```python
from build123d import *

# Parameters (mm, degrees)
BOSS_EXTRUDE1_DEPTH       = 5
M3X0_5_TAPPED_HOLE1_D     = 2.5
M3X0_5_TAPPED_HOLE1_DEPTH = 3
M3X0_5_TAPPED_HOLE1_TIP   = 0.751075774
BOSS_EXTRUDE2_DEPTH       = 5
CUT_EXTRUDE1_DEPTH        = 6
BOSS_EXTRUDE3_DEPTH       = 5
SKETCH12_W                = 42.426406872
SKETCH12_H                = 0.46
BOSS_EXTRUDE4_DEPTH       = 5
SKETCH13_W                = 0.46
SKETCH13_H                = 42.886406871
BOSS_EXTRUDE5_DEPTH       = 5
M2X0_4_TAPPED_HOLE1_D     = 1.6
SKETCH20_W                = 42.886406872
SKETCH20_H                = 1.7
CUT_EXTRUDE2_DEPTH        = 6
M3X0_5_TAPPED_HOLE3_D     = 2.5
M3X0_5_TAPPED_HOLE3_DEPTH = 6
M3X0_5_TAPPED_HOLE3_TIP   = 0.751075774


with BuildPart() as part:
    # Sketch2 → Boss-Extrude1 (new body)
    with BuildSketch(Plane.XY):
        Polygon((-19.445436483, 19.445436483), (26.516504294, -26.516504294), (-19.445436483, -26.516504294), align=None)
    extrude(amount=BOSS_EXTRUDE1_DEPTH)

    # M3x0.5 Tapped Hole1
    with Locations(Plane(origin=(0, 0, 0), x_dir=(0, 0, -1), z_dir=(0.707106781, 0.707106781, 0))):
        with Locations((-2.75, 19.75), (-2.75, -29.75)):
            Hole(M3X0_5_TAPPED_HOLE1_D / 2, depth=M3X0_5_TAPPED_HOLE1_DEPTH)
            with Locations((0, 0, -(M3X0_5_TAPPED_HOLE1_DEPTH + M3X0_5_TAPPED_HOLE1_TIP / 2))):  # 118° drill point
                Cone(0, M3X0_5_TAPPED_HOLE1_D / 2, M3X0_5_TAPPED_HOLE1_TIP, mode=Mode.SUBTRACT)

    # Sketch6 → Boss-Extrude2 (add, through all)
    with BuildSketch(Plane.XY.offset(5)):
        Polygon((-19.445436483, 19.445436483), (-15.909902577, 15.909902577), (-14.495689014, 17.324116139), (-18.03122292, 20.859650045), align=None)
        Polygon((26.516504294, -26.516504294), (22.980970389, -22.980970389), (24.395183951, -21.566756826), (27.930717857, -25.102290732), align=None)
    extrude(amount=-BOSS_EXTRUDE2_DEPTH)

    # Sketch7 → Cut-Extrude1 (cut, through all)
    with BuildSketch(Plane.XY.offset(5)):
        Polygon((-18.03122292, 20.859650045), (-14.495689014, 17.324116139), (-19.445436483, 12.374368671), (-19.445436483, 19.445436483), align=None)
        Polygon((24.395183951, -21.566756826), (19.445436483, -26.516504294), (26.516504294, -26.516504294), (27.930717857, -25.102290732), align=None)
    extrude(amount=-CUT_EXTRUDE1_DEPTH, mode=Mode.SUBTRACT)

    # Sketch11 → Boss-Extrude3 (add, through all)
    with BuildSketch(Plane(origin=(0, 0, 0), x_dir=(-1, 0, 0), z_dir=(0, 0, -1))):
        Polygon((-19.445436483, -26.516504294), (-22.980970389, -26.516504294), (-22.980970389, -22.980970389), align=None)
        Polygon((19.445436483, 12.374368671), (19.445436483, 15.909902577), (15.909902577, 15.909902577), align=None)
    extrude(amount=-BOSS_EXTRUDE3_DEPTH)

    # Sketch12 → Boss-Extrude4 (add, through all)
    with BuildSketch(Plane.XY.offset(5)):
        with Locations((1.767766953, -26.746504294)):
            Rectangle(SKETCH12_W, SKETCH12_H)
    extrude(amount=-BOSS_EXTRUDE4_DEPTH)

    # Sketch13 → Boss-Extrude5 (add, through all)
    with BuildSketch(Plane.XY.offset(5)):
        with Locations((-19.675436483, -5.533300859)):
            Rectangle(SKETCH13_W, SKETCH13_H)
    extrude(amount=-BOSS_EXTRUDE5_DEPTH)

    # M2x0.4 Tapped Hole1 (through all)
    with Locations(Plane(origin=(0, 0, 0), x_dir=(-1, 0, 0), z_dir=(0, 0, -1))):
        with Locations((17.905436483, -11.976504294), (17.905436483, -21.976504294)):
            Hole(M2X0_4_TAPPED_HOLE1_D / 2)

    # Sketch20 → Cut-Extrude2 (cut, through all)
    with BuildSketch(Plane.XY.offset(5)):
        with Locations((1.537766953, -26.126504294)):
            Rectangle(SKETCH20_W, SKETCH20_H)
    extrude(amount=-CUT_EXTRUDE2_DEPTH, mode=Mode.SUBTRACT)

    # M3x0.5 Tapped Hole3
    with Locations(Plane(origin=(0, -25.276504294, 0), x_dir=(-1, 0, 0), z_dir=(0, -1, 0))):
        with Locations((7.905436483, -2.5), (-7.094563517, -2.5)):
            Hole(M3X0_5_TAPPED_HOLE3_D / 2, depth=M3X0_5_TAPPED_HOLE3_DEPTH)
            with Locations((0, 0, -(M3X0_5_TAPPED_HOLE3_DEPTH + M3X0_5_TAPPED_HOLE3_TIP / 2))):  # 118° drill point
                Cone(0, M3X0_5_TAPPED_HOLE3_D / 2, M3X0_5_TAPPED_HOLE3_TIP, mode=Mode.SUBTRACT)


solid = part.part
```
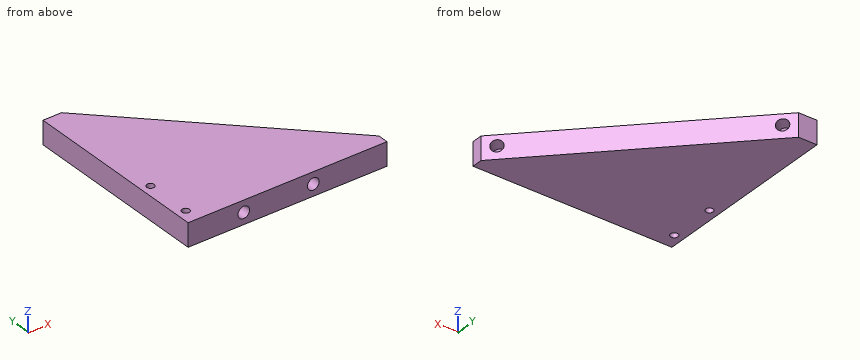
Read the model definition and answer for the solid it produces. Units are mm, in the model's axes. Coordinates: 2 decimals unless noted, no trailing zeros. Order: outer loops, then holes, each group sorted by start corner. A loop starts at its lowest first (then second) coordinate and runs counter-clockwise, first axis right, second up. Notation, with made-up numbers: (69.5, 41) - (77.5, 41) arc R15 cw to (77.5, 52) - close; hole circle Ø6 at (-38.5, 38.5). An arc over 180 degrees is marked (long way). Answer as a JSON object with one key per item and string values. Group by question number.
Item 1: Section B-B (y = -3) is taken. Give the vertices of the cut face in (x, z).
Item 2: Section A-A (z = 0.6) is taken. Give the vertices of the cut face in (x, y), plus the area to 3 significant figures.
Item 3: Consider probe 1 along Y at (x, z) = (-18, 2.5); probe 2 along X at (y, z) = (-12.5, 4.25); probe 3 along X at (y, z) = (7.5, 1). Determine where each line is inside the solid, lowest interval first. Write a range as from..to.
Item 4: Flat-ended cylindrical pins translate along their axes: P1, Ø2, axis at x = 7.09, z = 2.5, coming from the -Y side; P2, Ø3, axis at x = -7.91, z = 2.5, coming from the +Y side. Find the tip coordinate at first contact, or state that the pin passes through.
Item 5: Section C-C (x = 0.5) is taken. Give the vertices of the cut face in (y, z).
Results are:
{
 "1": {"outline": "(-19.91, 0) - (3, 0) - (3, 5) - (-19.91, 5) - close"},
 "2": {"outline": "(-19.91, -25.28) - (22.98, -25.28) - (22.98, -22.98) - (-15.91, 15.91) - (-19.91, 15.91) - close; hole circle Ø1.6 at (-17.91, -21.98); hole circle Ø1.6 at (-17.91, -11.98)", "area": "1,010 mm^2"},
 "3": {"probe 1": "y = -25.28..-22.77, -21.18..-12.77, -11.18..15.91", "probe 2": "x = -19.91..-18.51, -17.3..12.5", "probe 3": "x = -19.91..-7.5"},
 "4": {"P1": "stops at y = -19.13", "P2": "stops at y = 9.41"},
 "5": {"outline": "(-25.28, 0) - (-0.5, 0) - (-0.5, 5) - (-25.28, 5) - close"}
}
